Work out the finished part from the listing and answer in its coordinate system (mm). Face numbers are marked on the shaded views. A direction names the side the tool comes from. Round coordinates to 2 decimals unless told otherwise and drop trailing zeros. Order: outer loops, then holes, each group sorted by start corner. A loop starts at its lowest first (then second) coordinate and runs counter-clockwise, first axis right, second up. Notation, with made-up numbers: (36, 14) -> (50, 14) arc R21 cw to (50, 38) -> close; hole circle Ø11 at (-23, 26). An arc over 180 degrees is marked (long way). Use one line per item in the form item = value.
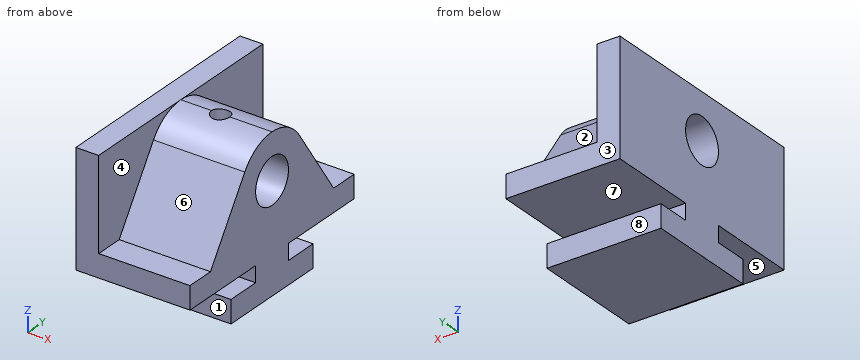
```python
from build123d import *

# Parameters (mm, degrees)
F0_R     = 12.7
F1_DEPTH = 50.8
F2_DEPTH = 12.7
F3_R     = 5.08
F4_DEPTH = 13.7612578348
F5_ANGLE = 90


with BuildPart() as f1:
    # F0 (on Front) → F1 (new body)
    with BuildSketch(Plane.XZ):
        with BuildLine():
            Line((31.75, 12.7), (31.75, 0))
            Line((31.75, 0), (95.25, 0))
            Line((95.25, 0), (95.25, 12.7))
            Line((95.25, 12.7), (76.2, 12.7))
            Line((76.2, 12.7), (76.2, 21.59))
            Line((76.2, 21.59), (127, 21.59))
            Line((127, 21.59), (127, 34.29))
            Line((127, 34.29), (111.125, 34.29))
            Line((111.125, 34.29), (84.5934256055, 73.8401730104))
            ThreePointArc((84.5934256055, 73.8401730104), (75.4529411765, 82.1017647059), (63.5, 85.09))
            ThreePointArc((63.5, 85.09), (51.5470588235, 82.1017647059), (42.4065743945, 73.8401730104))
            Line((42.4065743945, 73.8401730104), (15.875, 34.29))
            Line((15.875, 34.29), (0, 34.29))
            Line((0, 34.29), (0, 21.59))
            Line((0, 21.59), (50.8, 21.59))
            Line((50.8, 21.59), (50.8, 12.7))
            Line((50.8, 12.7), (31.75, 12.7))
        make_face()
        with Locations((63.5, 59.69)):
            Circle(F0_R, mode=Mode.SUBTRACT)
    extrude(amount=F1_DEPTH)

    # F0 (on Front) → F2 (join)
    with BuildSketch(Plane.XZ):
        with BuildLine():
            Line((31.75, 12.7), (31.75, 0))
            Line((31.75, 0), (95.25, 0))
            Line((95.25, 0), (95.25, 12.7))
            Line((95.25, 12.7), (76.2, 12.7))
            Line((76.2, 12.7), (76.2, 21.59))
            Line((76.2, 21.59), (127, 21.59))
            Line((127, 21.59), (127, 34.29))
            Line((127, 34.29), (111.125, 34.29))
            Line((111.125, 34.29), (84.5934256055, 73.8401730104))
            ThreePointArc((84.5934256055, 73.8401730104), (75.4529411765, 82.1017647059), (63.5, 85.09))
            ThreePointArc((63.5, 85.09), (51.5470588235, 82.1017647059), (42.4065743945, 73.8401730104))
            Line((42.4065743945, 73.8401730104), (15.875, 34.29))
            Line((15.875, 34.29), (0, 34.29))
            Line((0, 34.29), (0, 21.59))
            Line((0, 21.59), (50.8, 21.59))
            Line((50.8, 21.59), (50.8, 12.7))
            Line((50.8, 12.7), (31.75, 12.7))
        make_face()
        with Locations((63.5, 59.69)):
            Circle(F0_R, mode=Mode.SUBTRACT)
        with BuildLine():
            Line((0, 85.09), (0, 34.29))
            Line((0, 34.29), (15.875, 34.29))
            Line((15.875, 34.29), (42.4065743945, 73.8401730104))
            ThreePointArc((42.4065743945, 73.8401730104), (51.5470588235, 82.1017647059), (63.5, 85.09))
            Line((63.5, 85.09), (0, 85.09))
        make_face()
        with BuildLine():
            Line((111.125, 34.29), (127, 34.29))
            Line((127, 34.29), (127, 85.09))
            Line((127, 85.09), (63.5, 85.09))
            ThreePointArc((63.5, 85.09), (75.4529411765, 82.1017647059), (84.5934256055, 73.8401730104))
            Line((84.5934256055, 73.8401730104), (111.125, 34.29))
        make_face()
    extrude(amount=-F2_DEPTH)

    # F3 (on face) → F4 (cut, through all)
    with BuildSketch(Plane.XY.offset(85.09)):
        with Locations((63.5, -22.225)):
            Circle(F3_R)
    extrude(amount=-F4_DEPTH, mode=Mode.SUBTRACT)


with BuildPart() as f1_1:
    # F5: moved
    add(f1.part.rotate(Axis((0, 0, 59.69), (0, 0, 1)), F5_ANGLE))


solid = f1_1.part
```
Item 1: The part is cut by section C-C, the plane y = 14.5. Give the vertices of the cut face in (x, z), and give its area (3 significant figures).
Findings:
outline = (-12.7, 21.59) -> (50.8, 21.59) -> (50.8, 34.29) -> (0, 34.29) -> (0, 85.09) -> (-12.7, 85.09) -> close
area = 1,450 mm^2
Item 2: The part is cut by section D-D, the plane z = 44.5. Give the vertices of the cut face in (x, y), and give its area (3 significant figures).
Findings:
outline = (-12.7, 0) -> (0, 0) -> (0, 22.72) -> (50.8, 22.72) -> (50.8, 104.28) -> (0, 104.28) -> (0, 127) -> (-12.7, 127) -> close
area = 5,760 mm^2
Item 3: For the marked faces 1, 2, 3, 4 and 5, determine the directions among +Z, -Z, +X, -X, +Y, -Y from which every point of the face is accessible in a straight line to the end or side of a thin tool.
Findings:
face_1 = -Z, +X, -X, -Y
face_2 = +Z, +X, +Y
face_3 = +Z, -Z, +X, -X, +Y
face_4 = +Z, +X, -Y
face_5 = +X, -X, -Y
Item 4: Determine the mould class of the marked faces 6, 7 and 8 for opening direction Z: released by +Z, released by -Z, zero draft, split by the parting line, or undercut.
Findings:
face_6 = released by +Z
face_7 = undercut
face_8 = zero draft
Item 5: The part is cut by section A-A, the plane x = 9. Give the vertices of the cut face in (y, z) (3 decimals), and give its area (3 significant figures).
Findings:
outline = (0, 21.59) -> (50.8, 21.59) -> (50.8, 12.7) -> (31.75, 12.7) -> (31.75, 0) -> (95.25, 0) -> (95.25, 12.7) -> (76.2, 12.7) -> (76.2, 21.59) -> (127, 21.59) -> (127, 34.29) -> (111.125, 34.29) -> (84.593, 73.84) arc R25.4 ccw to (42.407, 73.84) -> (15.875, 34.29) -> (0, 34.29) -> close; hole circle Ø25.4 at (63.5, 59.69)
area = 5,190 mm^2
Item 6: The part is cut by section B-B, the plane z = 59.69. Give the vertices of the cut face in (x, y).
Findings:
outline = (-12.7, 0) -> (0, 0) -> (0, 32.91) -> (50.8, 32.91) -> (50.8, 50.8) -> (-12.7, 50.8) -> close; (-12.7, 76.2) -> (50.8, 76.2) -> (50.8, 94.09) -> (0, 94.09) -> (0, 127) -> (-12.7, 127) -> close
Item 7: Flat-ended cylindrical pins translate along their axes: P1, Ø17.5, axis at x = 29, y = 7.5, coming from the +Z side; P2, Ø8, axis at x = 13.5, z = 12.5, coming from the +Y side; P3, Ø12.5, axis at x = 33, y = 120, coming from the +Z side; P4, Ø20.5, axis at y = 63.5, z = 59.69, coming from the +X side. Find the tip coordinate at first contact, or state that the pin passes through.
Findings:
P1 = 34.85
P2 = 95.25
P3 = 34.29
P4 = through
Item 8: Consider line 1 along X through (y, z) = (63.5, 77.25) (3 decimals); line 2 along Z through (x, y) = (7, 63.5); line 3 along Y through (x, z) = (-3, 60.5). Determine where each line is inside the solid, lowest interval first.
Findings:
line_1 = -12.7 to 17.145, 27.305 to 50.8
line_2 = 0 to 46.99, 72.39 to 85.09
line_3 = 0 to 50.83, 76.17 to 127
